Here's how the part is built. I have some questions about the finished solid (model axes, mm). Face numbers are marked on the shaded views. A direction names the side the tool comes from. Coordinates: 2 decimals unless noted, no trailing zeros. Write each loop counter-clockwise with the first axis right and the second up, starting at its lowest first coordinate (ties: lowest second). Pieces come first, ordered by that corner, then holes. Notation, with made-up numbers: M 7,62 L 60,62 A32 ccw 60,94 Z; hole C 79,80 d9. An arc over 180 degrees is marked long. Write each question's results on one line, items separated by ' | '. Start each with the question number.
from build123d import *

# Parameters (mm, degrees)
SKETCH_1_W      = 20
SKETCH_1_H      = 10.6
SKETCH_1_R      = 1.1
EXTRUDE_1_DEPTH = 3.2
SKETCH_3_W      = 0.4
SKETCH_3_H      = 3.1
EXTRUDE_2_DEPTH = 3.5
EXTRUDE_3_DEPTH = 2
SKETCH_5_R      = 2.3
EXTRUDE_4_DEPTH = 1.9


with BuildPart() as part:
    # 草图1 → 凸台-拉伸1 (new body, symmetric)
    with BuildSketch(Plane(origin=(0, 0, 0), x_dir=(1, 0, 0), z_dir=(0, 1, 0))):
        Rectangle(SKETCH_1_W, SKETCH_1_H)
        with Locations((-4.8, -2.3)):
            Circle(SKETCH_1_R, mode=Mode.SUBTRACT)
        with Locations((4.8, -2.3)):
            Circle(SKETCH_1_R, mode=Mode.SUBTRACT)
    extrude(amount=EXTRUDE_1_DEPTH, both=True)

    # 草图3 → 凸台-拉伸2 (add)
    with BuildSketch(Plane.XY.offset(5.3)):
        with Locations((-8.1, 0)):
            Rectangle(SKETCH_3_W, SKETCH_3_H)
        with Locations((-0.7, 0)):
            Rectangle(SKETCH_3_W, SKETCH_3_H)
        with Locations((8.3, 0)):
            Rectangle(SKETCH_3_W, SKETCH_3_H)
    extrude(amount=EXTRUDE_2_DEPTH)

    # 草图4 → 凸台-拉伸3 (add, symmetric)
    with BuildSketch(Plane(origin=(0, 0, 0), x_dir=(1, 0, 0), z_dir=(0, 1, 0))):
        with BuildLine():
            Line((6.3, 4.662469082), (6.3, 5.863134893))
            Line((6.3, 5.863134893), (-11.464883061, 10.1))
            Line((-11.464883061, 10.1), (-10.444126954, 14.379959926))
            ThreePointArc((-10.444126954, 14.379959926), (-8.335887623, 15.676234173), (-7.039613376, 13.567994841))
            Line((-7.039613376, 13.567994841), (-7.990772476, 9.579850364))
            Line((-7.990772476, 9.579850364), (6.6, 6.1))
            Line((6.6, 6.1), (6.6, 4.662469082))
            Line((6.6, 4.662469082), (6.3, 4.662469082))
        make_face()
    extrude(amount=EXTRUDE_3_DEPTH, both=True)

    # 草图5 → 凸台-拉伸4 (add, symmetric)
    with BuildSketch(Plane(origin=(0, 0, 0), x_dir=(1, 0, 0), z_dir=(0, 1, 0))):
        with Locations((-8.741870165, 13.973977384)):
            Circle(SKETCH_5_R)
    extrude(amount=EXTRUDE_4_DEPTH, both=True)


solid = part.part
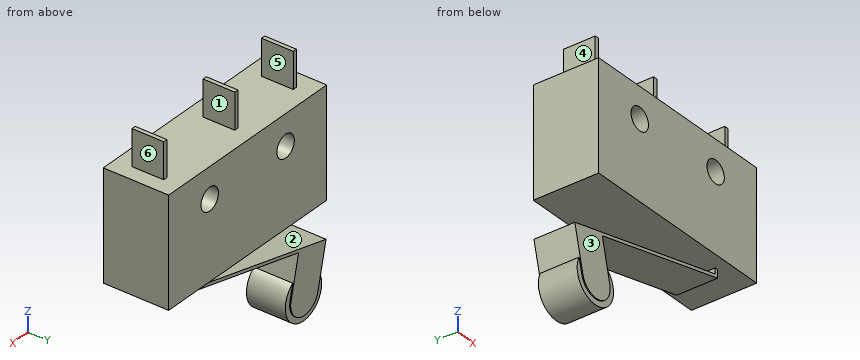
1) For pin 1 Ø5 at (x, z) = (-3.5, -8.5) entering from +Y; pin 2 Ø0.9 at (y, z) = (-0.5, 7.5) entering from -X; pin 3 Ø0.9 at (y, z) = (0.5, 6.5) entering from +X; pin 4 Ø1.8 at (x, z) = (-4.8, 2.3) entering from -Y, each with a flat end and sliding along its axis, tell me the tip position at first contact or that it passes through.
2) I want a section at C-C, the plane y = -0.5. Write out the boundary of the cut face in (x, z).
3) We'd pull the mould along Z, two halves only. Please class the marked faces 1 and 2: pulls with the +Z half, pulls with the -Z half, needs draft (parallel to the pull), parting line crosses it, or undercut.
4) I want a section at B-B, the plane x = 4.8. Write out the boundary of the cut face in (y, z), then the cut area to 3 significant figures.
5) I want a section at D-D, the plane x = 7.5. Write out the boundary of the cut face in (y, z), then the cut area to 3 significant figures.
6) Please list where these lines run through material, in increasing order: line 1 (X direction, y = -1, z = 2.3); line 2 (X direction, y = 1.5, z = 7.5); line 3 (Z direction, x = 4.8, y = -0.5). Write a range as [from, to].
7) For the marked faces 3, 4, 5 and 6, which set-ups out of +Z, -Z, +X, -X, +Y, -Y let a thin tool reach every point of the face, with its end or its side?
8) I want a section at A-A, the plane z = 2.3. Write out the boundary of the cut face in (x, y), then the cut area to 3 significant figures.
Output:
1) pin 1: stops at y = 2 | pin 2: stops at x = -8.3 | pin 3: stops at x = 8.5 | pin 4: passes through
2) outline: M -11.46,-10.1 L -10.79,-12.93 A2.3 ccw long -7.39,-12.12 L -7.99,-9.58 L 6.6,-6.1 L 6.6,-5.3 L 10,-5.3 L 10,5.3 L 8.5,5.3 L 8.5,8.8 L 8.1,8.8 L 8.1,5.3 L -0.5,5.3 L -0.5,8.8 L -0.9,8.8 L -0.9,5.3 L -7.9,5.3 L -7.9,8.8 L -8.3,8.8 L -8.3,5.3 L -10,5.3 L -10,-5.3 L 6.3,-5.3 L 6.3,-5.86 Z; hole C -4.8,2.3 d2.2; hole C 4.8,2.3 d2.2
3) face 1: needs draft | face 2: undercut
4) outline: M -3.2,-5.3 L 3.2,-5.3 L 3.2,1.2 L -3.2,1.2 Z; M -3.2,3.4 L 3.2,3.4 L 3.2,5.3 L -3.2,5.3 Z; M -2,-6.53 L 2,-6.53 L 2,-6.22 L -2,-6.22 Z | area: 55.0 mm2
5) outline: M -3.2,-5.3 L 3.2,-5.3 L 3.2,5.3 L -3.2,5.3 Z | area: 67.8 mm2
6) line 1: x = [-10, -5.9], [-3.7, 3.7], [5.9, 10] | line 2: x = [-8.3, -7.9], [-0.9, -0.5], [8.1, 8.5] | line 3: z = [-6.53, -6.22], [-5.3, 1.2], [3.4, 5.3]
7) face 3: -Z, +X, -X, -Y | face 4: +Z, -X, +Y, -Y | face 5: +Z, +Y, -Y | face 6: +Z, +X, +Y, -Y
8) outline: M -10,-3.2 L -5.9,-3.2 L -5.9,3.2 L -10,3.2 Z; M -3.7,-3.2 L 3.7,-3.2 L 3.7,3.2 L -3.7,3.2 Z; M 5.9,-3.2 L 10,-3.2 L 10,3.2 L 5.9,3.2 Z | area: 99.8 mm2
